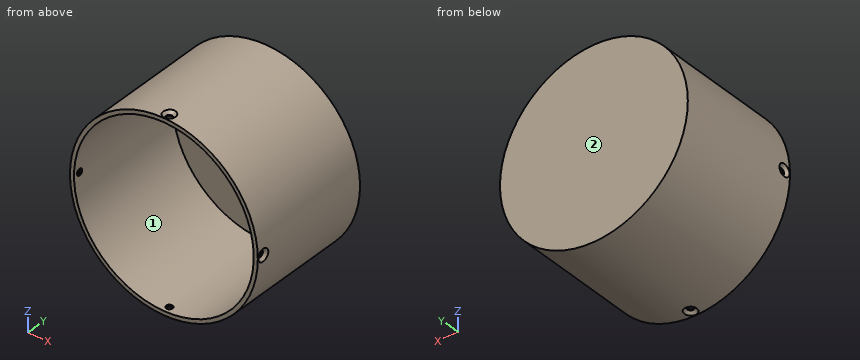
from build123d import *

# Parameters (mm, degrees)
SKETCH3_R           = 23.075
BOSS_EXTRUDE3_DEPTH = 31.6
SKETCH4_R           = 22.075
CUT_EXTRUDE1_DEPTH  = 30.6
CIRPATTERN1_COUNT   = 4


# Read off the part's stored shape, not the designer's step: CSK for M2 Flat Head Machine Screw2
with BuildPart() as part:
    # Sketch3 → Boss-Extrude3 (new body)
    with BuildSketch(Plane(origin=(0, 0, 0), x_dir=(1, 0, 0), z_dir=(0, 1, 0))):
        with Locations(Location((0, 0, 0), (0, 0, 270))):
            Circle(SKETCH3_R)
    extrude(amount=BOSS_EXTRUDE3_DEPTH)

    # Sketch4 → Cut-Extrude1 (cut)
    with BuildSketch(Plane.XZ):
        with Locations(Location((0, 0, 0), (0, 0, 270))):
            Circle(SKETCH4_R)
    extrude(amount=-CUT_EXTRUDE1_DEPTH, mode=Mode.SUBTRACT)

    # CSK for M2 Flat Head Machine Screw2 outl → CSK for M2 Flat Head Machine Screw2 (revolve, cut)
    with BuildSketch(Plane(origin=(0, 1.7, 0), x_dir=(0, 1, 0), z_dir=(0, 0, -1))):
        Polygon((1.550011104, 23.075011104), (0, 23.075011104), (0, 22.060491405), (0.8, 22.060491405), (0.8, 22.325), align=None)
    csk_for_m2_flat_head_machine_screw2 = revolve(axis=Axis((0, 1.7, 0), (1, 0, 0)), mode=Mode.SUBTRACT)

    # CirPattern1: CSK for M2 Flat Head Machine Screw2 ×4 about axis
    cirpattern1_axis = Axis((0, 30.6, 0), (0, -1, 0))
    for i in range(1, CIRPATTERN1_COUNT):
        add(csk_for_m2_flat_head_machine_screw2.rotate(cirpattern1_axis, i * 360 / CIRPATTERN1_COUNT), mode=Mode.SUBTRACT)


solid = part.part
Verification items for the finished model (mm, model axes). Face numbers are marked on the shaded views. A direction names the side the tool comes from. Give positions to 0.01 mm unless a question says otherwise; leave off trailing zeros. Write each loop counter-clockwise with the first axis right and the second up, starting at its lowest first coordinate (ties: lowest second). Pieces come first, ordered by that corner, then holes. Notation, with made-up numbers: M 81,56 L 135,56 A21 cw 135,77 Z; hole C 33.5,-25.5 d9. An arc over 180 degrees is marked long. Write item = value, one per line.
(1) Material ranges on line 1 (X direction, y = 22, z = 0) (3 decimals); line 2 (Y direction, x = 0, z = -22.15); line 3 (Y direction, x = 0, z = -22), recorded low to high.
Found:
line_1 = -23.075 to -22.075, 22.075 to 23.075
line_2 = 0 to 0.9, 2.5 to 31.6
line_3 = 30.6 to 31.6
(2) Sectioned sample at C-C (y = 1.7). Give the number of separate pieces and of enclosed holes in the cut face, then the cut area to 3 significant figures.
Found:
separate_pieces = 4
enclosed_holes = 0
area = 133 mm2
(3) Go/stop test with flat-tipped pins: pin 1 Ø1.5 at (x, y) = (-11.5, 9) entering from +Z; pin 2 Ø2 at (x, z) = (0.5, -9) entering from -Y; pin 3 Ø2.5 at (y, z) = (1.7, 0) entering from -X (3 decimals); pin 4 Ø1.3 at (y, z) = (1.7, 0) entering from +X. Record where each tip stops, or that it passes through.
Found:
pin_1 = 20.42
pin_2 = 30.6
pin_3 = -22.775
pin_4 = through
(4) Sectioned sample at D-D (z = 7). Record the cut outline in (x, y), then the cut area to 3 significant figures.
Found:
outline = M -21.99,0 L -20.94,0 L -20.94,30.6 L 20.94,30.6 L 20.94,0 L 21.99,0 L 21.99,31.6 L -21.99,31.6 Z
area = 108 mm2
(5) Access from +Z, -Z, +X, -X, +Y, -Y to the whole of each face (thin tool, end or side, straight path). Record for the marked faces 1 and 2.
Found:
face_1 = -Y
face_2 = +Z, -Z, +X, -X, +Y
(6) Sectioned sample at A-A (z = 0). Record the cut outline in (x, y) (3 decimals), then the cut area to 3 significant figures.
Found:
outline = M -23.075,0 L -22.075,0 L -22.075,0.9 L -22.325,0.9 L -23.075,0.15 Z; M -23.075,3.25 L -22.325,2.5 L -22.075,2.5 L -22.075,30.6 L 22.075,30.6 L 22.075,2.5 L 22.325,2.5 L 23.075,3.25 L 23.075,31.6 L -23.075,31.6 Z; M 22.075,0 L 23.075,0 L 23.075,0.15 L 22.325,0.9 L 22.075,0.9 Z
area = 103 mm2
(7) Sectioned sample at B-B (x = 0). Record the cut outline in (y, z) (3 decimals), then the cut area to 3 significant figures.
Found:
outline = M 0,-23.075 L 0.15,-23.075 L 0.9,-22.325 L 0.9,-22.075 L 0,-22.075 Z; M 0,22.075 L 0.9,22.075 L 0.9,22.325 L 0.15,23.075 L 0,23.075 Z; M 2.5,-22.325 L 3.25,-23.075 L 31.6,-23.075 L 31.6,23.075 L 3.25,23.075 L 2.5,22.325 L 2.5,22.075 L 30.6,22.075 L 30.6,-22.075 L 2.5,-22.075 Z
area = 103 mm2
